from build123d import *

# Parameters (mm, degrees)
BOSS_EXTRUDE1_DEPTH = 60
SKETCH2_R           = 1.5
BOSS_EXTRUDE2_DEPTH = 4
SKETCH3_R           = 1.5
BOSS_EXTRUDE3_DEPTH = 4


with BuildPart() as part:
    # Sketch1 → Boss-Extrude1 (new body)
    with BuildSketch(Plane.XY):
        Polygon((-0.918598934, -3.331524887), (2.081401066, -1.599474079), (2.081401066, 1.864627536), (-0.918598934, 3.596678344), (-3.918598934, 1.864627536), (-3.918598934, -1.599474079), align=None)
    extrude(amount=BOSS_EXTRUDE1_DEPTH)

    # Sketch2 → Boss-Extrude2 (add)
    with BuildSketch(Plane.XY.offset(60)):
        with Locations((-0.918598934, 0.132576728)):
            Circle(SKETCH2_R)
    extrude(amount=BOSS_EXTRUDE2_DEPTH)

    # Sketch3 → Boss-Extrude3 (add)
    with BuildSketch(Plane(origin=(0, 0, 0), x_dir=(-1, 0, 0), z_dir=(0, 0, -1))):
        with Locations((0.918598934, 0.132576728)):
            Circle(SKETCH3_R)
    extrude(amount=BOSS_EXTRUDE3_DEPTH)


solid = part.part
Geometry: final body of the model. Coordinates: model frame, mm. A direction names the side the tool comes from. Coordinates: 2 decimals unless noted, no trailing zeros. Order: outer loops, then holes, each group sorted by start corner. A loop starts at its lowest first (then second) coordinate and runs counter-clockwise, first axis right, second up.
1) Ray query, probe 1 along Z at (x, y) = (0.5, 1.25); probe 2 along Y at (x, z) = (-0.75, 21); probe 3 along Y at (x, z) = (-0.5, 42.5) (3 decimals). Return the intervals inside material, ascending.
Result sheet:
probe 1: z = 0 to 60
probe 2: y = -3.23 to 3.5
probe 3: y = -3.09 to 3.355
2) Section B-B (z = 53). Return loops of the section in (x, y), then the cut area to 3 significant figures.
Result sheet:
outline: (-3.92, -1.6) - (-0.92, -3.33) - (2.08, -1.6) - (2.08, 1.86) - (-0.92, 3.6) - (-3.92, 1.86) - close
area: 31.2 mm2
3) Section C-C (x = 0). Return loops of the section in (y, z).
Result sheet:
outline: (-2.8, 0) - (-1.05, 0) - (-1.05, -4) - (1.32, -4) - (1.32, 0) - (3.07, 0) - (3.07, 60) - (1.32, 60) - (1.32, 64) - (-1.05, 64) - (-1.05, 60) - (-2.8, 60) - close
4) Set-up query: faces 1 (the flat face through (-2.4, 2.74, 29.58)), 2 (the flat face through (-1.6, -1.4, 60)), 3 (the flat face through (-1.6, -1.4, 0)). Return all of +Z, -Z, +X, -X, +Y, -Y with unobstructed straight access to the full face (end or side cutting, diameter ignored); none if empty.
Result sheet:
face 1: +Z, -Z, -X, +Y
face 2: +Z
face 3: -Z
5) First-contact query: P1, Ø1, axis at x = -2.5, y = -2, coming from the -Z side; P2, Ø1.5, axis at x = -3, z = 26.5, coming from the +Y side. Flat tips, straight axial feed; report the tip coordinate or a pass-through.
Result sheet:
P1: stops at z = 0
P2: stops at y = 2.83
6) Section A-A (y = 0.75). Return loops of the section in (x, z).
Result sheet:
outline: (-3.92, 0) - (-2.29, 0) - (-2.29, -4) - (0.45, -4) - (0.45, 0) - (2.08, 0) - (2.08, 60) - (0.45, 60) - (0.45, 64) - (-2.29, 64) - (-2.29, 60) - (-3.92, 60) - close
7) Section D-D (y = -2.75). Return loops of the section in (x, z), then the cut area to 3 significant figures.
Result sheet:
outline: (-1.93, 0) - (0.09, 0) - (0.09, 60) - (-1.93, 60) - close
area: 121 mm2
